Source: CAD feature listing. Evaluate the final solid. Frame: model axes, mm. A direction names the side the tool comes from. Coordinates: 2 decimals unless noted, no trailing zeros. Loops run counter-clockwise (first coordinate to the right, second up) from the corner with the lowest first, then second, coordinate; pieces in that order, holes last.
Item 1: Section query D-D, the plane x = 2. Return the cut outline in (y, z), then the cut area to 3 significant figures.
Item 2: Section query C-C, the plane x = -5.5. Return the cut outline in (y, z), then the cut area to 3 significant figures.
Item 3: Line query: probe 1 along Y at (x, z) = (10.5, -21.05); probe 2 along X at (y, z) = (-4, -4); probe 3 along Y at (x, z) = (-18.85, -14.5). Output: solid intervals per line, ascending.
Item 4: Pin query (flat end, axial travel): pin 1 Ø1 at (y, z) = (0, -19) entering from +X; pin 2 Ø1.2 at (y, z) = (-6, -16.5) entering from -X; pin 3 Ø4.5 at (x, y) = (-10.5, -7) entering from +Z. Return the tip coordinate at first contact, or that it passes through.
Item 5: Pull-direction query (X, two-part tool) for faces 5 (the flat face through (-0.053, -7.627, -18.472)), 6 (the cylindrical face through (-22.03, -0.03, -19.63)), 7 (the flat face through (-18.5, 1, -4)); classes: +X half, -X half, draft (parallel to the pull), parting line (faces both ways), or undercut.
Item 6: Section query B-B, the plane z = -12.5. Return the cut outline in (x, y), then the cut area to 3 significant figures.
Item 7: Reachability of faces 1 (the flat face through (17, 4, -20)), 2 (the cylindrical face through (2.339, 6.623, -19.564)), 3 (the cylindrical face through (-2.339, 6.623, -19.564)), 4 (the cylindrical face through (-22, 4, -19)) from +Z, -Z, +X, -X, +Y, -Y: full face, straight path, thin tool, end or side. Return the list, or none.
Item 8: Section query A-A, the plane z = -4.5. Return the cut outline in (x, y).
```python
from build123d import *

# Parameters (mm, degrees)
BOSS_EXTRU_1_DEPTH      = 5
ESQUISSE4_W             = 2.5
ESQUISSE4_H             = 5
ENL_V_MAT_EXTRU_1_DEPTH = 7.5
ENL_V_MAT_EXTRU_2_REACH = 51.497
ESQUISSE5_R             = 1
CONG_1_R                = 2.5
CONG_2_R                = 5
ESQUISSE6_W             = 26
ESQUISSE6_H             = 18.5
ESQUISSE6_R             = 0.91
BOSS_EXTRU_2_DEPTH      = 3
NERVURE4_REACH          = 35.479
ESQUISSE7_WALL_W        = 74.793384568
ESQUISSE7_WALL_H        = 2.5
NERVURE5_REACH          = 35.479
ESQUISSE8_WALL_W        = 78.919505224
ESQUISSE8_WALL_H        = 2.5
CONG_3_R                = 2.5
CONG_4_START            = -2.015218214
CONG_4_3_DEPTH          = 4.030436428
CONG_4_START_2          = 3.7499999
CONG_4_4_DEPTH          = 1.2500001
CONG_4_START_3          = -5
CONG_4_5_DEPTH          = 1.25
CONG_4_6_DEPTH          = 10
ENL_V_MAT_EXTRU_3_REACH = 53.377
ESQUISSE9_R             = 0.95


with BuildPart() as part:
    # Esquisse2 → Boss.-Extru.1 (new, symmetric)
    with BuildSketch(Plane(origin=(0, 0, 0), x_dir=(1, 0, 0), z_dir=(0, 1, 0))):
        Polygon((-18.5, -5), (-18.5, 16), (18.5, 16), (18.5, -5), (22.5, -5), (22.5, 20), (-22.5, 20), (-22.5, -5), align=None)
    extrude(amount=BOSS_EXTRU_1_DEPTH, both=True)

    # Esquisse4 → Enlèv. mat.-Extru.1 (cut)
    with BuildSketch(Plane(origin=(0, 5, 0), x_dir=(1, 0, 0), z_dir=(0, 1, 0))):
        with Locations((20.5, 0)):
            Rectangle(ESQUISSE4_W, ESQUISSE4_H)
    extrude(amount=-ENL_V_MAT_EXTRU_1_DEPTH, mode=Mode.SUBTRACT)

    # Enlèv. mat.-Extru.2: up to this face of the body (flat: up to its plane)
    enl_v_mat_extru_2_end = Plane(part.part.faces().sort_by_distance((18.5, 0, -5.5))[0])
    # Esquisse5 → Enlèv. mat.-Extru.2 (cut, up to the picked face)
    with BuildSketch(Plane(origin=(22.5, 0, 0), x_dir=(0, 0, -1), z_dir=(1, 0, 0)), mode=Mode.PRIVATE) as enl_v_mat_extru_2_sk1:
        Circle(ESQUISSE5_R)
    enl_v_mat_extru_2_tool1 = split(extrude(enl_v_mat_extru_2_sk1.sketch, amount=-ENL_V_MAT_EXTRU_2_REACH, mode=Mode.PRIVATE), bisect_by=enl_v_mat_extru_2_end, keep=Keep.BOTH, mode=Mode.PRIVATE)
    add(enl_v_mat_extru_2_tool1.solids().sort_by(Axis((22.5, 0, 0), (-1, 0, 0)))[0], mode=Mode.SUBTRACT)

    # Congé1
    cong_1_edges = [part.edges().sort_by_distance(p)[0] for p in [
        (20.5, -2.5, 2.5),
        (20.5, -2.5, -2.5),
    ]]
    fillet(cong_1_edges, radius=CONG_1_R - 0.0001)  # a hair under: the kernel refuses the full size

    # Congé2
    # the kernel refuses this fillet: 5 mm, written as the material it takes off along each edge
    with BuildSketch(Plane(origin=(-35, -5, 5), x_dir=(0, 1, 0), z_dir=(1, 0, 0)), Plane(origin=(-35, 5, 5), x_dir=(0, 0, -1), z_dir=(1, 0, 0)), Plane(origin=(6, -5, 5), x_dir=(0, 1, 0), z_dir=(1, 0, 0)), Plane(origin=(6, 5, 5), x_dir=(0, 0, -1), z_dir=(1, 0, 0))) as cong_2_piece_1:
        with BuildLine():
            CenterArc((CONG_2_R, -CONG_2_R), CONG_2_R, 90, 90)
            Line((0, -CONG_2_R), (0, 0))
            Line((0, 0), (CONG_2_R, 0))
        make_face()
    extrude(amount=29, mode=Mode.SUBTRACT)

    # Esquisse6 → Boss.-Extru.2 (add)
    with BuildSketch(Plane(origin=(0, 0, -20), x_dir=(-1, 0, 0), z_dir=(0, 0, -1))):
        Rectangle(ESQUISSE6_W, ESQUISSE6_H)
        with Locations((-10.5, 6.75)):
            Circle(ESQUISSE6_R, mode=Mode.SUBTRACT)
        with Locations((10.5, 6.75)):
            Circle(ESQUISSE6_R, mode=Mode.SUBTRACT)
        with Locations((10.5, -6.75)):
            Circle(ESQUISSE6_R, mode=Mode.SUBTRACT)
        with Locations((-10.5, -6.75)):
            Circle(ESQUISSE6_R, mode=Mode.SUBTRACT)
    extrude(amount=BOSS_EXTRU_2_DEPTH)

    # Esquisse7 wall → Nervure4 (add, up to next)
    with BuildSketch(Plane(origin=(0, 7.125, -18), x_dir=(0, -0.728199992693, 0.685364699005), z_dir=(0, -0.685364699005, -0.728199992693)), mode=Mode.PRIVATE) as nervure4_sk1:
        Rectangle(ESQUISSE7_WALL_W, ESQUISSE7_WALL_H)
    nervure4_tool1 = extrude(nervure4_sk1.sketch, amount=NERVURE4_REACH, mode=Mode.PRIVATE) - part.part
    nervure4 = nervure4_tool1.solids().sort_by_distance((0, 7.125, -18))[0]
    add(nervure4)

    # Symétrie1: Nervure4 across plane
    add(nervure4.mirror(Plane.ZX))

    # Esquisse8 wall → Nervure5 (add, up to next)
    with BuildSketch(Plane(origin=(17.75, 0, -21.5), x_dir=(0.953582665134, 0, 0.301131367937), z_dir=(0.301131367937, 0, -0.953582665134)), mode=Mode.PRIVATE) as nervure5_sk1:
        Rectangle(ESQUISSE8_WALL_W, ESQUISSE8_WALL_H)
    nervure5_tool1 = extrude(nervure5_sk1.sketch, amount=-NERVURE5_REACH, mode=Mode.PRIVATE) - part.part
    nervure5 = nervure5_tool1.solids().sort_by_distance((17.75, 0, -21.5))[0]
    add(nervure5)

    # Symétrie2: Nervure5 across plane
    add(nervure5.mirror(Plane(origin=(0, 0, 0), x_dir=(0, 0, 1), z_dir=(1, 0, 0))))

    # Congé3
    cong_3_edges = [part.edges().sort_by_distance(p)[0] for p in [
        (1.25, 7.125, -20),
        (-1.25, 7.125, -20),
        (-1.25, -7.125, -20),
        (1.25, -7.125, -20),
        (17.75, 1.25, -20),
        (17.75, -1.25, -20),
        (-17.75, -1.25, -20),
        (-17.75, 1.25, -20),
        (-13, -9.25, -21.5),
        (-13, 9.25, -21.5),
        (13, 9.25, -21.5),
        (13, -9.25, -21.5),
    ]]
    fillet(cong_3_edges, radius=CONG_3_R)

    # Congé4: read off the stored shape, not the designer's step
    # Congé4 outline → Congé4 (revolve, cut)
    with BuildSketch(Plane(origin=(0, 3.75, -22.5), x_dir=(0, 1, 0), z_dir=(0, 0, -1))):
        with BuildLine():
            Line((2.5, 22.5), (2.5, 20))
            ThreePointArc((2.5, 20), (3.232233047, 21.767766953), (5, 22.5))
            Line((5, 22.5), (2.5, 22.5))
        make_face()
        with BuildLine():
            ThreePointArc((5, -22.5), (3.232233047, -21.767766953), (2.5, -20))
            Line((2.5, -20), (2.5, -22.5))
            Line((2.5, -22.5), (5, -22.5))
        make_face()
    revolve(axis=Axis((0, 3.75, -22.5), (1, 0, 0)), mode=Mode.SUBTRACT)

    # Cong_4 2 outline → Cong_4 2 (revolve, cut)
    with BuildSketch(Plane(origin=(0, -3.75, -22.5), x_dir=(0, 1, 0), z_dir=(0, 0, -1))):
        with BuildLine():
            Line((2.5, 22.5), (2.5, 20))
            ThreePointArc((2.5, 20), (3.232233047, 21.767766953), (5, 22.5))
            Line((5, 22.5), (2.5, 22.5))
        make_face()
        with BuildLine():
            ThreePointArc((5, -22.5), (3.232233047, -21.767766953), (2.5, -20))
            Line((2.5, -20), (2.5, -22.5))
            Line((2.5, -22.5), (5, -22.5))
        make_face()
    revolve(axis=Axis((0, -3.75, -22.5), (1, 0, 0)), mode=Mode.SUBTRACT)

    # Cong_4 3 outline → Cong_4 3 (cut)
    with BuildSketch(Plane(origin=(0, 0, 0), x_dir=(1, 0, 0), z_dir=(0, 1, 0)).offset(CONG_4_START)):
        with BuildLine():
            Line((22.5, 18.167781731), (22.5, 15.999999998))
            Line((22.5, 15.999999998), (24, 15.999999998))
            Line((24, 15.999999998), (24, 19.52631579))
            Line((24, 19.52631579), (22.449089048, 20.016077143))
            Line((22.449089048, 20.016077143), (20.75282842, 20.551738394))
            ThreePointArc((20.75282842, 20.551738394), (22.016441302, 19.645605968), (22.5, 18.167781731))
        make_face()
        with BuildLine():
            Line((-24, 15.999999998), (-22.5, 15.999999998))
            Line((-22.5, 15.999999998), (-22.5, 18.167781731))
            ThreePointArc((-22.5, 18.167781731), (-22.016441302, 19.645605968), (-20.75282842, 20.551738394))
            Line((-20.75282842, 20.551738394), (-22.449089048, 20.016077143))
            Line((-22.449089048, 20.016077143), (-24, 19.52631579))
            Line((-24, 19.52631579), (-24, 15.999999998))
        make_face()
    extrude(amount=CONG_4_3_DEPTH, mode=Mode.SUBTRACT)

    # Cong_4 4 outline → Cong_4 4 (cut)
    with BuildSketch(Plane(origin=(0, 0, 0), x_dir=(1, 0, 0), z_dir=(0, 1, 0)).offset(CONG_4_START_2)):
        with BuildLine():
            Line((18.5, 20), (20, 20))
            ThreePointArc((20, 20), (21.767766953, 19.267766953), (22.5, 17.5))
            Line((22.5, 17.5), (22.5, 18.167781731))
            ThreePointArc((22.5, 18.167781731), (22.016441302, 19.645605968), (20.75282842, 20.551738394))
            Line((20.75282842, 20.551738394), (18.5, 21.263157895))
            Line((18.5, 21.263157895), (18.5, 20))
        make_face()
        with BuildLine():
            Line((-18.5, 20), (-18.5, 21.263157895))
            Line((-18.5, 21.263157895), (-20.75282842, 20.551738394))
            ThreePointArc((-20.75282842, 20.551738394), (-22.016441302, 19.645605968), (-22.5, 18.167781731))
            Line((-22.5, 18.167781731), (-22.5, 17.5))
            ThreePointArc((-22.5, 17.5), (-21.767766953, 19.267766953), (-20, 20))
            Line((-20, 20), (-18.5, 20))
        make_face()
    extrude(amount=CONG_4_4_DEPTH, mode=Mode.SUBTRACT)

    # Cong_4 5 outline → Cong_4 5 (cut)
    with BuildSketch(Plane(origin=(0, 0, 0), x_dir=(1, 0, 0), z_dir=(0, 1, 0)).offset(CONG_4_START_3)):
        with BuildLine():
            Line((18.5, 20), (20, 20))
            ThreePointArc((20, 20), (21.767766953, 19.267766953), (22.5, 17.5))
            Line((22.5, 17.5), (22.5, 18.167781731))
            ThreePointArc((22.5, 18.167781731), (22.016441302, 19.645605968), (20.75282842, 20.551738394))
            Line((20.75282842, 20.551738394), (18.5, 21.263157895))
            Line((18.5, 21.263157895), (18.5, 20))
        make_face()
        with BuildLine():
            Line((-18.5, 20), (-18.5, 21.263157895))
            Line((-18.5, 21.263157895), (-20.75282842, 20.551738394))
            ThreePointArc((-20.75282842, 20.551738394), (-22.016441302, 19.645605968), (-22.5, 18.167781731))
            Line((-22.5, 18.167781731), (-22.5, 17.5))
            ThreePointArc((-22.5, 17.5), (-21.767766953, 19.267766953), (-20, 20))
            Line((-20, 20), (-18.5, 20))
        make_face()
    extrude(amount=CONG_4_5_DEPTH, mode=Mode.SUBTRACT)

    # Cong_4 6 outline → Cong_4 6 (add)
    with BuildSketch(Plane(origin=(0, 0, 0), x_dir=(1, 0, 0), z_dir=(0, 1, 0)).offset(CONG_4_START_3)):
        with BuildLine():
            Line((18.5, 13.5), (18.5, 16))
            Line((18.5, 16), (16, 16))
            ThreePointArc((16, 16), (17.767766953, 15.267766953), (18.5, 13.5))
        make_face()
        with BuildLine():
            ThreePointArc((-18.5, 13.5), (-17.767766953, 15.267766953), (-16, 16))
            Line((-16, 16), (-18.5, 15.999999998))
            Line((-18.5, 15.999999998), (-18.5, 13.5))
        make_face()
    extrude(amount=CONG_4_6_DEPTH)

    # Esquisse9 → Enlèv. mat.-Extru.3 (cut, up to next)
    with BuildSketch(Plane.ZY.offset(22.5), mode=Mode.PRIVATE) as enl_v_mat_extru_3_sk1:
        with Locations((-4.5, 0)):
            Circle(ESQUISSE9_R)
    enl_v_mat_extru_3_tool1 = extrude(enl_v_mat_extru_3_sk1.sketch, amount=-ENL_V_MAT_EXTRU_3_REACH, mode=Mode.PRIVATE) & part.part
    # Esquisse9 → Enlèv. mat.-Extru.3 (cut, up to next)
    with BuildSketch(Plane.ZY.offset(22.5), mode=Mode.PRIVATE) as enl_v_mat_extru_3_sk2:
        with Locations((-14.5, 0)):
            Circle(ESQUISSE9_R)
    enl_v_mat_extru_3_tool2 = extrude(enl_v_mat_extru_3_sk2.sketch, amount=-ENL_V_MAT_EXTRU_3_REACH, mode=Mode.PRIVATE) & part.part
    add(enl_v_mat_extru_3_tool1.solids().sort_by_distance((-22.5, 0, -4.5))[0], mode=Mode.SUBTRACT)
    add(enl_v_mat_extru_3_tool2.solids().sort_by_distance((-22.5, 0, -14.5))[0], mode=Mode.SUBTRACT)


solid = part.part
```
Verdict:
1. outline: (-9.25, -23) - (9.25, -23) - (9.25, -20) - (8.49, -19.29) - (5, -19.29) - (5, -16) - (-5, -16) - (-5, -19.29) - (-8.49, -19.29) - (-9.25, -20) - close
1. area: 101 mm2
2. outline: (-9.25, -23) - (9.25, -23) - (9.25, -20) - (5, -20) - (5, -16) - (-5, -16) - (-5, -20) - (-9.25, -20) - close
2. area: 95.5 mm2
3. probe 1: y = -9.25 to -7.66, -5.84 to 5.84, 7.66 to 9.25
3. probe 2: x = -22.5 to -18.5, 18.5 to 22.5
3. probe 3: y = -5 to -0.95, 0.95 to 5
4. pin 1: stops at x = 22.48
4. pin 2: stops at x = -1.25
4. pin 3: stops at z = -16
5. face 5: draft
5. face 6: -X half
5. face 7: undercut
6. outline: (-22.5, -5) - (-18.5, -5) - (-18.5, 5) - (-22.5, 5) - close; (18.5, -5) - (22.5, -5) - (22.5, 5) - (18.5, 5) - close
6. area: 80.0 mm2
7. face 1: -Z, +X, +Y
7. face 2: +Z, +X, +Y
7. face 3: +Z, -X, +Y
7. face 4: -Z, -X, +Y
8. outline: (-22.5, -5) - (-18.5, -5) - (-18.5, -0.95) - (-22.5, -0.95) - close; (-22.5, 0.95) - (-18.5, 0.95) - (-18.5, 5) - (-22.5, 5) - close; (18.5, -5) - (22.5, -5) - (22.5, 5) - (18.5, 5) - close
